Model file for the job. Use its own axes, mm. Give positions to 0.01 mm unless a question says otherwise; leave off trailing zeros. Loops run counter-clockwise (first coordinate to the right, second up) from the corner with the lowest first, then second, coordinate; pieces in that order, holes last. Notation, with made-up numbers: (-9, 72.5) -> (34, 72.5) arc R21 ccw to (34, 80.5) -> close; hole circle Ø2 at (-13.5, 2). An arc over 180 degrees is marked (long way). Use CSV: the item, a comma, the result in double quotes. Start each with the question number.
(1) Flat gauge pins, fed straight in: pin 1 (2 mm diameter, centred on x = 22, z = 23, fed in from +Y); pin 2 (8 mm diameter, centred on x = 11, z = 4.5, fed in from -Y); pin 3 (1.5 mm diameter, centred on x = 8, z = 29.5, fed in from -Y). Where does each tip first touch, or does it go through?
(2) Cut at A-A on z = 34.5. Write the cut outline in (x, y), then the cut area to 3 significant figures.
(3) Drill centre lines: probe 1 along Y at (x, z) = (46.5, 7); probe 2 along Y at (x, z) = (7, 10); probe 3 along X at (y, z) = (524.5, 20.5). Where is each one in solid material? Low to high.
(4) Cut at B-B on x = 41. Write the cut outline in (y, z), then the cut area to 3 significant figures.
from build123d import *

# Parameters (mm, degrees)
ESQUISSE1_W                  = 50
ESQUISSE1_H                  = 550
BOSS_EXTRU_1_DEPTH           = 40
BOSS_EXTRU_2_DEPTH           = 40
ENL_V_MAT_EXTRU_1_DEPTH      = 554.714727996
ENL_V_MAT_EXTRU_1_DEPTH_BACK = 554.714727996


with BuildPart() as part:
    # Esquisse1 → Boss.-Extru.1 (new body)
    with BuildSketch(Plane.XY):
        with Locations((25, 275)):
            Rectangle(ESQUISSE1_W, ESQUISSE1_H)
    extrude(amount=BOSS_EXTRU_1_DEPTH)

    # Esquisse2 → Boss.-Extru.2 (add)
    with BuildSketch(Plane.XY.offset(40)):
        Polygon((50, 0), (0, 0), (0, -28.867513459), align=None)
    extrude(amount=-BOSS_EXTRU_2_DEPTH)

    # Esquisse3 → Enlèv. mat.-Extru.1 (cut, two sides: drawn at the far end of the back side and taken through both)
    with BuildSketch(Plane.XY.offset(40).offset(-ENL_V_MAT_EXTRU_1_DEPTH_BACK)):
        Polygon((50, 521.132486541), (0, 550), (50, 550), align=None)
    extrude(amount=ENL_V_MAT_EXTRU_1_DEPTH + ENL_V_MAT_EXTRU_1_DEPTH_BACK, mode=Mode.SUBTRACT)


solid = part.part
Check result:
1,pin 1,"y = 537.88"
1,pin 2,"y = -24.83"
1,pin 3,"y = -24.68"
2,outline,"(0, -28.87) -> (50, 0) -> (50, 521.13) -> (0, 550) -> close"
2,area,"27,500 mm²"
3,probe 1,"-2.02 to 523.15"
3,probe 2,"-24.83 to 545.96"
3,probe 3,"0 to 44.17"
4,outline,"(-5.2, 0) -> (526.33, 0) -> (526.33, 40) -> (-5.2, 40) -> close"
4,area,"21,300 mm²"
